from build123d import *

# Parameters (mm, degrees)
SKETCH_1_R               = 47.5
EXTRUDE_1_DEPTH          = 13
SKETCH_2_R               = 31
EXTRUDE_2_DEPTH          = 2
SKETCH_3_R               = 15
CUT_EXTRUDE_2_DEPTH      = 2
SKETCH_6_R               = 11.5
CUT_EXTRUDE_3_DEPTH      = 69.421487853
CHAMFER_1_SIZE           = 1
SKETCH_7_R               = 7
CUT_EXTRUDE_4_DEPTH      = 9
SKETCH_8_R               = 4.5
CUT_EXTRUDE_5_DEPTH      = 68.775364256
PATTERN_CIRCULAR_1_COUNT = 4
CHAMFER_2_SIZE           = 1


with BuildPart() as part:
    # 草图1 → 凸台-拉伸1 (new body)
    with BuildSketch(Plane.XY):
        with Locations(Location((0, 0, 0), (0, 0, 180))):
            Circle(SKETCH_1_R)
    extrude(amount=EXTRUDE_1_DEPTH)

    # 草图2 → 凸台-拉伸2 (add)
    with BuildSketch(Plane.XY.offset(13)):
        Circle(SKETCH_2_R)
    extrude(amount=EXTRUDE_2_DEPTH)

    # 草图3 → 切除-拉伸2 (cut)
    with BuildSketch(Plane.XY.offset(15)):
        Circle(SKETCH_3_R)
    extrude(amount=-CUT_EXTRUDE_2_DEPTH, mode=Mode.SUBTRACT)

    # 草图6 → 切除-拉伸3 (cut, through all)
    with BuildSketch(Plane.XY.offset(13)):
        Circle(SKETCH_6_R)
    extrude(amount=-CUT_EXTRUDE_3_DEPTH, mode=Mode.SUBTRACT)

    # 倒角1
    chamfer_1_edges = [part.edges().sort_by_distance(p)[0] for p in [
        (-11.5, 0, 0),
        (-11.5, 0, 13),
    ]]
    chamfer(chamfer_1_edges, length=CHAMFER_1_SIZE)

    # 草图7 → 切除-拉伸4 (cut)
    with BuildSketch(Plane(origin=(0, 0, 0), x_dir=(-1, 0, 0), z_dir=(0, 0, -1))):
        with Locations((0, 39)):
            Circle(SKETCH_7_R)
    cut_extrude_4 = extrude(amount=-CUT_EXTRUDE_4_DEPTH, mode=Mode.SUBTRACT)

    # 草图8 → 切除-拉伸5 (cut, through all)
    with BuildSketch(Plane(origin=(0, 0, 9), x_dir=(-1, 0, 0), z_dir=(0, 0, -1))):
        with Locations((0, 39)):
            Circle(SKETCH_8_R)
    cut_extrude_5 = extrude(amount=-CUT_EXTRUDE_5_DEPTH, mode=Mode.SUBTRACT)

    # 阵列(圆周)1: 切除-拉伸4, 切除-拉伸5 ×4 about axis
    pattern_circular_1_axis = Axis((0, 0, 0), (0, 0, 1))
    add([cut_extrude_4.rotate(pattern_circular_1_axis, i * 360 / PATTERN_CIRCULAR_1_COUNT) for i in range(1, PATTERN_CIRCULAR_1_COUNT)], mode=Mode.SUBTRACT)
    add([cut_extrude_5.rotate(pattern_circular_1_axis, i * 360 / PATTERN_CIRCULAR_1_COUNT) for i in range(1, PATTERN_CIRCULAR_1_COUNT)], mode=Mode.SUBTRACT)

    # 倒角2
    chamfer_2_edges = [part.edges().sort_by_distance(p)[0] for p in [
        (47.5, 0, 0),
    ]]
    chamfer(chamfer_2_edges, length=CHAMFER_2_SIZE)


solid = part.part
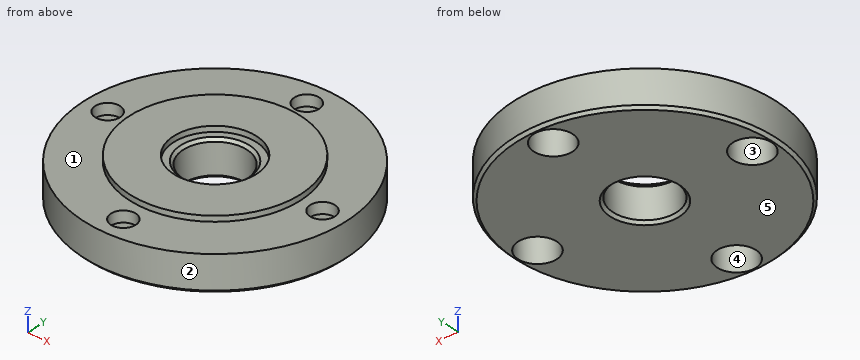
Could you check a few things on this model? Use its own coordinates, in mm. Face numbers are marked on the shaded views. A direction names the side the tool comes from. Round coordinates to 2 decimals unless told otherwise and drop trailing zeros. Loops run counter-clockwise (first coordinate to the right, second up) from the corner with the lowest first, then second, coordinate; pieces in that order, holes last. Notation, with made-up numbers: (64, 41) - (102, 41) arc R25 cw to (102, 69) - close; hole circle Ø5 at (-39, -39.75). An arc over 180 degrees is marked (long way). Write item = value, one per line.
1) I'm going to push flat-ended pins straight in: P1, Ø4, axis at x = -3, y = 41.5, coming from the -Z side; P2, Ø24, axis at x = 0.5, y = -2.5, coming from the +Z side; P3, Ø2, axis at y = -14, z = 13, coming from the -X side. Where does each tip first touch, or does it pass through?
Computed:
P1 = 9
P2 = 13
P3 = -45.69
2) Imagine slicing it at B-B (y = 0). Give the number of separate pieces and of enclosed holes in the cut face, and give its area (3 significant figures).
Computed:
separate_pieces = 4
enclosed_holes = 0
area = 673 mm2
3) On a 3-axis mill with a long thin cutter (end or side, diameter ignored), from which of +Z, -Z, +X, -X, +Y, -Y can I reach the whole of each face in a straight line? I mean the marked faces 4 and 5. Say none if no direction works.
Computed:
face_4 = -Z
face_5 = -Z, +X, -X, +Y, -Y
4) Imagine slicing it at A-A (z = 10.25). Please give me the cut outline in (x, y).
Computed:
outline = circle Ø95 at (0, 0); hole circle Ø9 at (-39, 0); hole circle Ø23 at (0, 0); hole circle Ø9 at (0, -39); hole circle Ø9 at (0, 39); hole circle Ø9 at (39, 0)
5) If we mould it in two halves opening along Y, with no side actions, what happens to the marked faces 1, 2 and 3? For each: pulls with the +Y half, pulls with the -Y half, needs draft (parallel to the pull), parting line crosses it, or undercut.
Computed:
face_1 = needs draft
face_2 = parting line crosses it
face_3 = undercut
6) I need wall thicknesses on line 1 along Y through (x, z) = (0, 10.15); line 2 along Y through (x, z) = (0, 7.25); line 3 along X through (y, z) = (-1, 8.5). Which ranges of each line are inside material? Lowest first, please. Write a range as from..to.
Computed:
line_1 = -47.5..-43.5, -34.5..-11.5, 11.5..34.5, 43.5..47.5
line_2 = -47.5..-46, -32..-11.5, 11.5..32, 46..47.5
line_3 = -47.49..-45.93, -32.07..-11.46, 11.46..32.07, 45.93..47.49
7) Imagine slicing it at C-C (z = 4.5). Please give me the cut outline in (x, y).
Computed:
outline = circle Ø95 at (0, 0); hole circle Ø14 at (-39, 0); hole circle Ø23 at (0, 0); hole circle Ø14 at (0, -39); hole circle Ø14 at (0, 39); hole circle Ø14 at (39, 0)
